Source: CAD feature listing. Evaluate the final solid. Frame: model axes, mm. Face numbers are marked on the shaded views. A direction names the side the tool comes from. Round coordinates to 2 decimals unless told otherwise and drop trailing zeros. Loops run counter-clockwise (first coordinate to the right, second up) from the corner with the lowest first, then second, coordinate; pieces in that order, holes last. Notation, with made-up numbers: (70, -36) -> (114, -36) arc R32 ccw to (114, -10) -> close; hole circle Ø4 at (-17.5, 15.25). An arc over 180 degrees is marked (long way). Write item = value, one per line.
from build123d import *

# Parameters (mm, degrees)
EXTRUDE1_DEPTH            = 53.34
LPATTERN1_COUNT           = 6
LPATTERN1_PITCH           = 10.16
LPATTERN1_COL_COUNT       = 6
LPATTERN1_COL_PITCH       = 10.16
F_4_CLEARANCE_HOLE2_D     = 3.2639
F_4_CLEARANCE_HOLE2_DEPTH = 15.24
F_4_CLEARANCE_HOLE2_TIP   = 0.980574487


with BuildPart() as part:
    # Sketch1 → Extrude1 (new, symmetric)
    with BuildSketch(Plane.XY):
        Polygon((0, 0), (0, 15.875), (1.5875, 15.875), (1.5875, 1.5875), (15.875, 1.5875), (15.875, 0), align=None)
    extrude(amount=EXTRUDE1_DEPTH, both=True)

    # Sketch3 → #4 Clearance Hole1 (revolve, cut)
    with BuildSketch(Plane(origin=(5.0419, 1.5875, 0), x_dir=(0, 0, 1), z_dir=(1, 0, 0))):
        Polygon((0, 0), (0, 16.220574487), (1.63195, 15.24), (1.63195, 0), align=None)
    f_4_clearance_hole1 = revolve(axis=Axis((5.0419, 7.9375, 0), (0, -1, 0)), mode=Mode.SUBTRACT)

    # LPattern1: #4 Clearance Hole1 ×6
    with Locations(*[(0, 0, i * LPATTERN1_PITCH) for i in range(1, LPATTERN1_COUNT)]):
        add(f_4_clearance_hole1, mode=Mode.SUBTRACT)

    # LPattern1 col: #4 Clearance Hole1 ×6
    with Locations(*[(0, 0, -i * LPATTERN1_COL_PITCH) for i in range(1, LPATTERN1_COL_COUNT)]):
        add(f_4_clearance_hole1, mode=Mode.SUBTRACT)

    # #4 Clearance Hole2
    with Locations(Plane(origin=(1.5875, 7.64032, -41.275), x_dir=(0, 1, 0), z_dir=(1, 0, 0))):
        with Locations((0, 0), (0, 82.55)):
            Hole(F_4_CLEARANCE_HOLE2_D / 2, depth=F_4_CLEARANCE_HOLE2_DEPTH)
            with Locations((0, 0, -(F_4_CLEARANCE_HOLE2_DEPTH + F_4_CLEARANCE_HOLE2_TIP / 2))):  # 118° drill point
                Cone(0, F_4_CLEARANCE_HOLE2_D / 2, F_4_CLEARANCE_HOLE2_TIP, mode=Mode.SUBTRACT)


solid = part.part
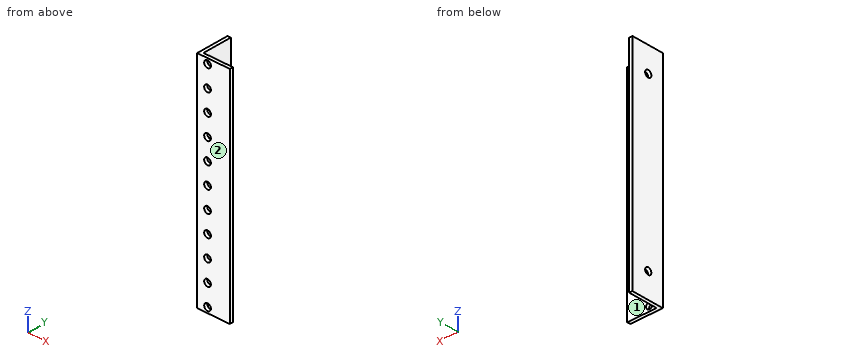
1. Section query B-B (z = -15.5). Return the cut outline in (x, y) (1 decimal), then the cut area to 3 significant figures.
Evaluation:
outline = (0, 0) -> (15.9, 0) -> (15.9, 1.6) -> (1.6, 1.6) -> (1.6, 15.9) -> (0, 15.9) -> close
area = 47.9 mm²
2. Section query A-A (z = 30.48). Return the cut outline in (x, y) (1 decimal).
Evaluation:
outline = (0, 0) -> (3.4, 0) -> (3.4, 1.6) -> (1.6, 1.6) -> (1.6, 15.9) -> (0, 15.9) -> close; (6.7, 0) -> (15.9, 0) -> (15.9, 1.6) -> (6.7, 1.6) -> close
3. Line query: probe 1 along Y at (x, z) = (9.75, 26.5); probe 2 along X at (y, z) = (0.7, 30.48) (3 decimals). Output: solid intervals per line, ascending. Write a range as from..to.
Evaluation:
probe_1 = 0..1.59
probe_2 = 0..3.41, 6.674..15.875
4. Contact query for flat-ended pins moving along their axis: pin 1 Ø4 at (x, z) = (5.04, -40.64) entering from -Y; pin 2 Ø3 at (x, z) = (5.04, -50.8) entering from -Y; pin 3 Ø4 at (y, z) = (7, -0.5) entering from +X; pin 4 Ø5 at (x, z) = (10.5, 36) entering from +Y. Output: stop coordinate, or through.
Evaluation:
pin_1 = 0
pin_2 = through
pin_3 = 1.59
pin_4 = 1.59
5. Section query C-C (x = 12.5). Return the cut outline in (y, z).
Evaluation:
outline = (0, -53.34) -> (1.59, -53.34) -> (1.59, 53.34) -> (0, 53.34) -> close
6. Set-up query: the marked faces 1 and 2. Return all of +Z, -Z, +X, -X, +Y, -Y with unobstructed straight access to the full face (end or side cutting, diameter ignored); none if empty.
Evaluation:
face_1 = +Z, -Z, +X, +Y
face_2 = +Z, -Z, +X, -X, -Y
